Can you work these out from the model? Positions are in its coordinate system, mm. A direction names the side the tool comes from. Give positions to 0.01 mm unless a question says otherwise; leave off trailing zeros. Loops run counter-clockwise (first coordinate to the right, second up) from the corner with the lowest first, then second, coordinate; pieces in that order, holes last. Notation, with made-up numbers: (52, -27) -> (98, -27) arc R28 cw to (98, -1) -> close; hole circle Ø6 at (82, 2). An arc over 180 degrees is marked (long way). Return JSON: item names as keys, results as strings. Group by question number.
Q1. Suppose I cut it at C-C, the plane z = 5.5. Please give me the cut outline in (x, y).
Q2. Will these pins go through, and if not, where does the flat tip stop? pin 1 (1.6 mm diameter, centred on y = 4.5, z = 15.5, fed in from +X); pin 2 (2 mm diameter, centred on x = 7, y = 21, fed in from -Z); pin 3 (2 mm diameter, centred on x = 22.5, y = 4.5, fed in from +Z).
Q3. Which directions (+Z, -Z, +X, -X, +Y, -Y) give clear straight access to the entire face, cutting with the end or side of a thin tool? Please do faces 1 (the flat face through (15, 7, 15)), 2 (the flat face through (5, 21, 2)), 3 (the flat face through (10, 5, 17)), 4 (the flat face through (5, 18, 1.5)).
Q4. Suppose I cut it at D-D, the plane y = 4.5. Please give me the cut outline in (x, z), and give its area (4 significant figures).
Q5. I need wall thicknesses on line 1 along X through (y, z) = (7.5, 16.5); line 2 along X through (y, z) = (1, 5.5); line 3 along X through (y, z) = (20.95, 6.5). Which ranges of each line are inside material? Lowest first, please. Write a range as [from, to].
Q6. Suppose I cut it at A-A, the plane y = 18.75. Please give me the cut outline in (x, z).
Q7. Suppose I cut it at B-B, the plane x = 14. Please give me the cut outline in (y, z).
Q8. Thinking about a two-plate mould opening in Y: for faces 5 (the flat face through (16, 9.5, 18)), 6 (the flat face through (15, 7, 12.5)), 7 (the flat face through (24, 3, 13)), which applies, pulls with the +Y half, pulls with the -Y half, needs draft (parallel to the pull), parting line crosses it, or undercut?
```python
from build123d import *

# Parameters (mm, degrees)
EXTRUDE_1_DEPTH          = 7
CUT_EXTRUDE_START        = -5
SKETCH_2_R               = 4
CUT_EXTRUDE_1_DEPTH      = 5
SKETCH_3_W               = 29.5
SKETCH_3_H               = 11
EXTRUDE_2_DEPTH          = 8
SKETCH_4_W               = 10.5
SKETCH_4_H               = 10
SKETCH_4_W_2             = 9
EXTRUDE_3_DEPTH          = 7
SKETCH_5_W               = 8
SKETCH_5_H               = 9
CUT_EXTRUDE_2_DEPTH      = 2
SKETCH_6_R               = 2.5
CUT_EXTRUDE_3_DEPTH      = 2.2
SKETCH_7_R               = 1.6
CUT_EXTRUDE_4_DEPTH      = 45.443784717
SKETCH_8_W               = 10
SKETCH_8_H               = 5
EXTRUDE_4_DEPTH          = 8
CUT_EXTRUDE_5_DEPTH      = 3
SKETCH_11_W              = 8
SKETCH_11_H              = 6.5
EXTRUDE_6_DEPTH          = 5
EXTRUDE_7_DEPTH          = 1
EXTRUDE_8_DEPTH          = 1
CUT_EXTRUDE_6_DEPTH      = 4
SKETCH_15_W              = 7
SKETCH_15_H              = 4.5
CUT_EXTRUDE_7_DEPTH      = 2
SKETCH_16_W              = 1
SKETCH_16_H              = 4
CUT_EXTRUDE_8_DEPTH      = 1
CUT_EXTRUDE_9_DEPTH      = 46.521972716
CUT_EXTRUDE_9_DEPTH_BACK = 46.521972716
SKETCH_17_W              = 8.500817713
SKETCH_17_H              = 8.67771192
SKETCH_17_W_2            = 8.381247082
SKETCH_17_H_2            = 10.001242217
SKETCH_18_W              = 9
SKETCH_18_H              = 9.010392854
EXTRUDE_9_DEPTH          = 3


# Read off the part's stored shape, not the designer's step: 圆顶1, 圆顶2
with BuildPart() as part:
    # 草图1 → 凸台-拉伸1 (new body)
    with BuildSketch(Plane(origin=(0, 0, 0), x_dir=(1, 0, 0), z_dir=(0, 1, 0))):
        with BuildLine():
            Line((0, 0), (29.5, 0))
            Line((29.5, 0), (29.5, -2.5))
            Line((29.5, -2.5), (33.5, -2.5))
            ThreePointArc((33.5, -2.5), (37.5, -6.5), (33.5, -10.5))
            Line((33.5, -10.5), (29.5, -10.5))
            Line((29.5, -10.5), (29.5, -13))
            Line((29.5, -13), (0, -13))
            Line((0, -13), (0, -10.5))
            Line((0, -10.5), (-4, -10.5))
            ThreePointArc((-4, -10.5), (-8, -6.5), (-4, -2.5))
            Line((-4, -2.5), (0, -2.5))
            Line((0, -2.5), (0, 0))
        make_face()
    extrude(amount=EXTRUDE_1_DEPTH)

    # 草图2 → 切除-拉伸1 (cut)
    with BuildSketch(Plane(origin=(0, 7, 0), x_dir=(1, 0, 0), z_dir=(0, 1, 0)).offset(CUT_EXTRUDE_START)):
        with Locations((-4, -6.5)):
            Circle(SKETCH_2_R)
        with Locations((33.5, -6.5)):
            Circle(SKETCH_2_R)
    extrude(amount=CUT_EXTRUDE_1_DEPTH, mode=Mode.SUBTRACT)

    # 草图3 → 凸台-拉伸2 (add)
    with BuildSketch(Plane(origin=(0, 7, 0), x_dir=(1, 0, 0), z_dir=(0, 1, 0))):
        with Locations((14.75, -6.5)):
            Rectangle(SKETCH_3_W, SKETCH_3_H)
    extrude(amount=EXTRUDE_2_DEPTH)

    # 草图4 → 凸台-拉伸3 (add)
    with BuildSketch(Plane(origin=(0, 15, 0), x_dir=(1, 0, 0), z_dir=(0, 1, 0))):
        with Locations((23.75, -6.5)):
            Rectangle(SKETCH_4_W, SKETCH_4_H)
        with Locations((5, -6.5)):
            Rectangle(SKETCH_4_W_2, SKETCH_4_H)
    extrude(amount=EXTRUDE_3_DEPTH)

    # 草图5 → 切除-拉伸2 (cut)
    with BuildSketch(Plane(origin=(0, 22, 0), x_dir=(1, 0, 0), z_dir=(0, 1, 0))):
        with Locations((5, -6.5)):
            Rectangle(SKETCH_5_W, SKETCH_5_H)
    extrude(amount=-CUT_EXTRUDE_2_DEPTH, mode=Mode.SUBTRACT)

    # 草图6 → 切除-拉伸3 (cut)
    with BuildSketch(Plane(origin=(0, 22, 0), x_dir=(1, 0, 0), z_dir=(0, 1, 0))):
        with Locations(Location((23.75, -6.5, 0), (0, 0, 270))):
            Circle(SKETCH_6_R)
        with Locations(Location((4.75, -6.5, 0), (0, 0, 270))):
            Circle(SKETCH_6_R)
    extrude(amount=-CUT_EXTRUDE_3_DEPTH, mode=Mode.SUBTRACT)

    # 圆顶1 outline → 圆顶1 (revolve)
    with BuildSketch(Plane(origin=(4.75, 0, 6.5), x_dir=(1, 0, 0), z_dir=(0, 0, 1))):
        with BuildLine():
            Line((0, 19.8), (2.500000001, 19.799999998))
            ThreePointArc((2.500000001, 19.799999998), (1.60078106, 21.238476323), (0, 21.8))
            Line((0, 21.8), (0, 19.8))
        make_face()
    revolve(axis=Axis((4.75, 0, 6.5), (0, 1, 0)))

    # 圆顶2 outline → 圆顶2 (revolve)
    with BuildSketch(Plane(origin=(23.75, 0, 6.5), x_dir=(1, 0, 0), z_dir=(0, 0, 1))):
        with BuildLine():
            Line((0, 19.8), (2.500000001, 19.799999997))
            ThreePointArc((2.500000001, 19.799999997), (1.60078106, 21.238476323), (0, 21.8))
            Line((0, 21.8), (0, 19.8))
        make_face()
    revolve(axis=Axis((23.75, 0, 6.5), (0, 1, 0)))

    # 草图7 → 切除-拉伸4 (cut, through all)
    with BuildSketch(Plane(origin=(0, 2, 0), x_dir=(1, 0, 0), z_dir=(0, 1, 0))):
        with Locations(Location((-4, -6.5, 0), (0, 0, 270))):
            Circle(SKETCH_7_R)
        with Locations(Location((33.5, -6.5, 0), (0, 0, 270))):
            Circle(SKETCH_7_R)
    extrude(amount=-CUT_EXTRUDE_4_DEPTH, mode=Mode.SUBTRACT)

    # 草图8 → 凸台-拉伸4 (add)
    with BuildSketch(Plane.XY.offset(13)):
        with Locations((14.75, 2.5)):
            Rectangle(SKETCH_8_W, SKETCH_8_H)
    extrude(amount=EXTRUDE_4_DEPTH)

    # 草图10 → 切除-拉伸5 (cut)
    with BuildSketch(Plane.XZ):
        Polygon((9.75, 21), (9.75, 12), (1, 12), (1, 1), (28.5, 1), (28.5, 12), (19.75, 12), (19.75, 21), align=None)
    extrude(amount=-CUT_EXTRUDE_5_DEPTH, mode=Mode.SUBTRACT)

    # 草图11 → 凸台-拉伸6 (add)
    with BuildSketch(Plane(origin=(0, 5, 0), x_dir=(1, 0, 0), z_dir=(0, 1, 0))):
        with Locations((14.75, -17.75)):
            Rectangle(SKETCH_11_W, SKETCH_11_H)
    extrude(amount=EXTRUDE_6_DEPTH)

    # 草图12 → 凸台-拉伸7 (add)
    with BuildSketch(Plane(origin=(18.75, 0, 0), x_dir=(0, 0, -1), z_dir=(1, 0, 0))):
        Polygon((-14.5, 8.832927064), (-13, 8.172497524), (-13, 5), (-14.5, 5), align=None)
    extrude(amount=-EXTRUDE_7_DEPTH)

    # 草图13 → 凸台-拉伸8 (add)
    with BuildSketch(Plane.ZY.offset(-10.75)):
        Polygon((14.5, 8.832927064), (13, 8.172497524), (13, 5), (14.5, 5), align=None)
    extrude(amount=-EXTRUDE_8_DEPTH)

    # 草图14 → 切除-拉伸6 (cut)
    with BuildSketch(Plane.XY.offset(21)):
        Polygon((11.25, 5), (18.25, 5), (18.25, 9.5), (15.355989936, 9.5), (15.355989936, 10), (13.355989936, 10), (13.355989936, 9.5), (11.25, 9.5), align=None)
    extrude(amount=-CUT_EXTRUDE_6_DEPTH, mode=Mode.SUBTRACT)

    # 草图15 → 切除-拉伸7 (cut)
    with BuildSketch(Plane.XY.offset(17)):
        with Locations((14.75, 7.25)):
            Rectangle(SKETCH_15_W, SKETCH_15_H)
    extrude(amount=-CUT_EXTRUDE_7_DEPTH, mode=Mode.SUBTRACT)

    # 草图16 → 切除-拉伸8 (cut)
    with BuildSketch(Plane(origin=(0, 10, 0), x_dir=(1, 0, 0), z_dir=(0, 1, 0))):
        with Locations((11.75, -16.5)):
            Rectangle(SKETCH_16_W, SKETCH_16_H)
        with Locations((17.75, -16.5)):
            Rectangle(SKETCH_16_W, SKETCH_16_H)
    extrude(amount=-CUT_EXTRUDE_8_DEPTH, mode=Mode.SUBTRACT)

    # 草图17 → 切除-拉伸9 (cut, two sides: drawn at the far end of the back side and taken through both)
    with BuildSketch(Plane(origin=(0, 15, 0), x_dir=(1, 0, 0), z_dir=(0, 1, 0)).offset(-CUT_EXTRUDE_9_DEPTH_BACK)):
        with Locations((33.750408857, -6.83885596)):
            Rectangle(SKETCH_17_W, SKETCH_17_H)
        with Locations((-4.190623541, -7.500621109)):
            Rectangle(SKETCH_17_W_2, SKETCH_17_H_2)
    extrude(amount=CUT_EXTRUDE_9_DEPTH + CUT_EXTRUDE_9_DEPTH_BACK, mode=Mode.SUBTRACT)

    # 草图18 → 凸台-拉伸9 (add)
    with BuildSketch(Plane(origin=(0, 15, 0), x_dir=(1, 0, 0), z_dir=(0, 1, 0))):
        with Locations((14, -6.5)):
            Rectangle(SKETCH_18_W, SKETCH_18_H)
    extrude(amount=EXTRUDE_9_DEPTH)


solid = part.part
```
Ans:
{
 "1": {"outline": "(0, 0) -> (1, 0) -> (1, 3) -> (28.5, 3) -> (28.5, 0) -> (29.5, 0) -> (29.5, 15) -> (29, 15) -> (29, 22) -> (26.04, 22) -> (26.04, 19.8) arc R2.36 ccw to (21.46, 19.8) -> (21.46, 22) -> (18.5, 22) -> (18.5, 18) -> (9.5, 18) -> (9.5, 22) -> (9, 22) -> (9, 20) -> (7.04, 20) -> (7.04, 19.8) arc R2.36 ccw to (2.46, 19.8) -> (2.46, 20) -> (1, 20) -> (1, 22) -> (0.5, 22) -> (0.5, 15) -> (0, 15) -> close"},
 "2": {"pin 1": "stops at x = 19.75", "pin 2": "stops at z = 1.5", "pin 3": "stops at z = 13"},
 "3": {"face 1": "+Z", "face 2": "+Y", "face 3": "+Z, -X, +Y", "face 4": "-Z, +X, -X, +Y"},
 "4": {"outline": "(0, 0) -> (29.5, 0) -> (29.5, 13) -> (19.75, 13) -> (19.75, 21) -> (9.75, 21) -> (9.75, 13) -> (0, 13) -> close", "area": "463.5 mm^2"},
 "5": {"line 1": "x = [10.75, 11.25], [18.25, 18.75]", "line 2": "x = [0, 1], [28.5, 29.5]", "line 3": "x = [0.5, 1], [2.84, 6.66], [9, 9.5], [18.5, 21.25], [21.84, 25.66], [26.25, 29]"},
 "6": {"outline": "(0.5, 1.5) -> (9.5, 1.5) -> (9.5, 11.5) -> (0.5, 11.5) -> close; (18.5, 1.5) -> (29, 1.5) -> (29, 11.5) -> (18.5, 11.5) -> close"},
 "7": {"outline": "(0, 0) -> (7, 0) -> (7, 1) -> (15, 1) -> (15, 1.99) -> (18, 1.99) -> (18, 11.01) -> (15, 11.01) -> (15, 12) -> (7, 12) -> (7, 13) -> (5, 13) -> (5, 14.5) -> (10, 14.5) -> (10, 17) -> (9.5, 17) -> (9.5, 15) -> (5, 15) -> (5, 21) -> (3, 21) -> (3, 1) -> (0, 1) -> close"},
 "8": {"face 5": "undercut", "face 6": "pulls with the +Y half", "face 7": "needs draft"}
}
